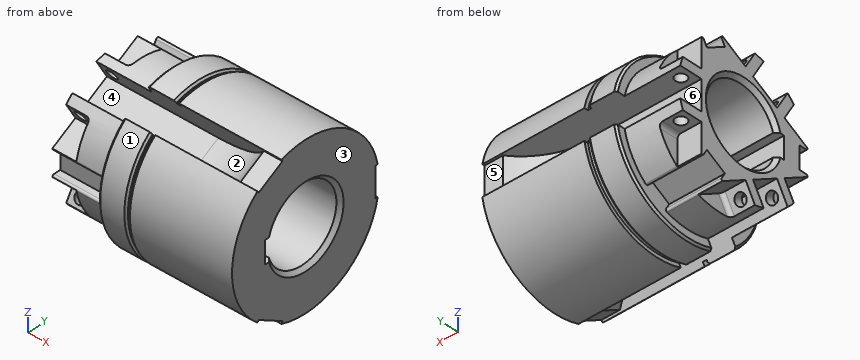
from build123d import *

# Parameters (mm, degrees)
CUT_EXTRUDE1_DEPTH       = 8
CIRPATTERN1_COUNT        = 3
CUT_EXTRUDE2_DEPTH       = 13
FILLET1_R                = 2
CUT_EXTRUDE3_REACH       = 125.655
SKETCH6_R                = 3
CIRPATTERN2_COUNT        = 3
FILLET1_OF_CIRPATTERN2_R = 2
CUT_EXTRUDE4_DEPTH       = 30
FILLET2_R                = 1
CIRPATTERN3_COUNT        = 3
FILLET2_OF_CIRPATTERN3_R = 1
CUT_EXTRUDE5_REACH       = 130.22
SKETCH9_W                = 102
SKETCH9_H                = 12
CHAMFER2_SIZE            = 2
CHAMFER3_SIZE            = 1


with BuildPart() as part:
    # Sketch1 → Revolve1 (revolve)
    with BuildSketch(Plane.XY, mode=Mode.PRIVATE) as revolve1_sk:
        Polygon((0, 20), (0, 42.5), (-55, 42.5), (-55, 40.5), (-57, 40.5), (-57, 42.5), (-72, 42.5), (-72, 37.6), (-102, 37.6), (-102, 20), align=None)
    revolve(revolve1_sk.sketch.rotate(Axis((-534.701035213, 0, 0), (1, 0, 0)), 90), axis=Axis((-534.701035213, 0, 0), (1, 0, 0)))

    # Sketch3 → Cut-Extrude1 (cut, symmetric)
    with BuildSketch(Plane.XY):
        with BuildLine():
            Line((-102, 24.5), (-42, 24.5))
            ThreePointArc((-42, 24.5), (-24.11145618, 28.72291236), (-10, 40.5))
            Line((-10, 40.5), (0, 40.5))
            Line((0, 40.5), (0, 42.5))
            Line((0, 42.5), (-55, 42.5))
            Line((-55, 42.5), (-55, 40.5))
            Line((-55, 40.5), (-57, 40.5))
            Line((-57, 40.5), (-57, 42.5))
            Line((-57, 42.5), (-72, 42.5))
            Line((-72, 42.5), (-72, 37.6))
            Line((-72, 37.6), (-102, 37.6))
            Line((-102, 37.6), (-102, 24.5))
        make_face()
    cut_extrude1 = extrude(amount=CUT_EXTRUDE1_DEPTH, both=True, mode=Mode.SUBTRACT)

    # CirPattern1: Cut-Extrude1 ×3 about axis
    cirpattern1_axis = Axis((0, 0, 0), (1, 0, 0))
    for i in range(1, CIRPATTERN1_COUNT):
        add(cut_extrude1.rotate(cirpattern1_axis, i * 360 / CIRPATTERN1_COUNT), mode=Mode.SUBTRACT)

    # Sketch4 → Cut-Extrude2 (cut)
    with BuildSketch(Plane.ZY.offset(102)):
        with BuildLine():
            Line((-13, 35.281156444), (-13, 24.5))
            Line((-13, 24.5), (-28.522096697, 24.5))
            ThreePointArc((-28.522096697, 24.5), (-21.449462979, 30.881718506), (-13, 35.281156444))
        make_face()
        with BuildLine():
            Line((13, 35.281156444), (13, 24.5))
            Line((13, 24.5), (28.522096697, 24.5))
            ThreePointArc((28.522096697, 24.5), (21.449462979, 30.881718506), (13, 35.281156444))
        make_face()
    cut_extrude2 = extrude(amount=-CUT_EXTRUDE2_DEPTH, mode=Mode.SUBTRACT)

    # Fillet1
    fillet1_edges = [part.edges().sort_by_distance(p)[0] for p in [
        (-89, 29.890578222, -13),
        (-89, 29.890578222, 13),
    ]]
    fillet(fillet1_edges, radius=FILLET1_R)

    # Cut-Extrude3: up to this face of the body (flat: up to its plane)
    cut_extrude3_end = Plane(part.part.faces().sort_by_distance((-96.5, 29.890578222, -13))[0])
    # Sketch6 → Cut-Extrude3 (cut, up to the picked face)
    with BuildSketch(Plane.XY.offset(13), mode=Mode.PRIVATE) as cut_extrude3_sk1:
        with Locations((-96.5, 30.5)):
            Circle(SKETCH6_R)
    cut_extrude3_tool1 = split(extrude(cut_extrude3_sk1.sketch, amount=-CUT_EXTRUDE3_REACH, mode=Mode.PRIVATE), bisect_by=cut_extrude3_end, keep=Keep.BOTH, mode=Mode.PRIVATE)
    cut_extrude3 = cut_extrude3_tool1.solids().sort_by(Axis((-96.5, 30.5, 13), (0, 0, -1)))[0]
    add(cut_extrude3, mode=Mode.SUBTRACT)

    # CirPattern2: Cut-Extrude2, Cut-Extrude3 ×3 about axis
    cirpattern2_axis = Axis((0, 0, 0), (1, 0, 0))
    add([cut_extrude2.rotate(cirpattern2_axis, i * 360 / CIRPATTERN2_COUNT) for i in range(1, CIRPATTERN2_COUNT)], mode=Mode.SUBTRACT)
    add([cut_extrude3.rotate(cirpattern2_axis, i * 360 / CIRPATTERN2_COUNT) for i in range(1, CIRPATTERN2_COUNT)], mode=Mode.SUBTRACT)

    # Fillet1 of CirPattern2
    fillet1_of_cirpattern2_edges = [part.edges().sort_by_distance(p)[0] for p in [
        (-89, -3.686958862, 32.386000074),
        (-89, -26.20361936, 19.386000074),
        (-89, -26.20361936, -19.386000074),
        (-89, -3.686958862, -32.386000074),
    ]]
    fillet(fillet1_of_cirpattern2_edges, radius=FILLET1_OF_CIRPATTERN2_R)

    # Sketch7 → Cut-Extrude4 (cut)
    with BuildSketch(Plane.ZY.offset(102)):
        with BuildLine():
            Line((-6, -37.118189611), (-6, -32.3))
            Line((-6, -32.3), (6, -32.3))
            Line((6, -32.3), (6, -37.118189611))
            ThreePointArc((6, -37.118189611), (0, -37.6), (-6, -37.118189611))
        make_face()
    cut_extrude4 = extrude(amount=-CUT_EXTRUDE4_DEPTH, mode=Mode.SUBTRACT)

    # Fillet2
    fillet2_edges = [part.edges().sort_by_distance(p)[0] for p in [
        (-87, -37.118189611, 6),
        (-87, -37.118189611, -6),
    ]]
    fillet(fillet2_edges, radius=FILLET2_R)

    # CirPattern3: Cut-Extrude4 ×3 about axis
    cirpattern3_axis = Axis((0, 0, 0), (1, 0, 0))
    for i in range(1, CIRPATTERN3_COUNT):
        add(cut_extrude4.rotate(cirpattern3_axis, i * 360 / CIRPATTERN3_COUNT), mode=Mode.SUBTRACT)

    # Fillet2 of CirPattern3
    fillet2_of_cirpattern3_edges = [part.edges().sort_by_distance(p)[0] for p in [
        (-87, 13.362942383, -35.145295146),
        (-87, 23.755247228, -29.145295146),
        (-87, 23.755247228, 29.145295146),
        (-87, 13.362942383, 35.145295146),
    ]]
    fillet(fillet2_of_cirpattern3_edges, radius=FILLET2_OF_CIRPATTERN3_R)

    # Sketch9 → Cut-Extrude5 (cut, up to next)
    with BuildSketch(Plane(origin=(0, -23.3, 0), x_dir=(1, 0, 0), z_dir=(0, 1, 0)), mode=Mode.PRIVATE) as cut_extrude5_sk1:
        with Locations((-51, 0)):
            Rectangle(SKETCH9_W, SKETCH9_H)
    cut_extrude5_tool1 = extrude(cut_extrude5_sk1.sketch, amount=CUT_EXTRUDE5_REACH, mode=Mode.PRIVATE) & part.part
    add(cut_extrude5_tool1.solids().sort_by_distance((-51, -23.3, 0))[0], mode=Mode.SUBTRACT)

    # Chamfer2
    chamfer2_edges = [part.edges().sort_by_distance(p)[0] for p in [
        (0, 20, 0),
        (-102, 20, 0),
    ]]
    chamfer(chamfer2_edges, length=CHAMFER2_SIZE)

    # Chamfer3
    chamfer3_edges = [part.edges().sort_by_distance(p)[0] for p in [
        (-72, -42.5, 0),
        (-72, 21.25, 36.806079661),
        (-57, -42.5, 0),
        (-57, 21.25, 36.806079661),
        (-72, 21.25, -36.806079661),
        (-57, 21.25, -36.806079661),
    ]]
    chamfer(chamfer3_edges, length=CHAMFER3_SIZE)


solid = part.part
The model under review builds one solid part; all positions refer to its coordinate system, in mm. Face numbers are marked on the shaded views. A direction names the side the tool comes from. Give positions to 0.01 mm unless a question says otherwise; leave off trailing zeros. Write each loop counter-clockwise with the first axis right and the second up, starting at its lowest first coordinate (ties: lowest second). Pieces come first, ordered by that corner, then holes. Notation, with made-up numbers: M -9.75,-2.75 L 24.25,-2.75 A31 cw 24.25,26.25 Z; hole C 86,25 d8. An arc over 180 degrees is marked long. One line per question, with ' | ' between items. Start each with the question number.
Item 1: Wall thickness on line 1 (Z direction, x = -60, y = 0); line 2 (Y direction, x = -96.5, z = -11.8); line 3 (Z direction, x = -24.5, y = -9): over which ranges is each line inside the solid? List them lowest first. Write a range as from..to.
Item 2: We need section A-A on z = 0. Write out the cut boundary in (x, y), plus the area to 3 significant figures.
Item 3: For the marked faces 4, 5 and 6, list the 3-axis set-ups (+Z, -Z, +X, -X, +Y, -Y) from which the entire face can be reached by the end or side of a thin tool; tool diameter is ignored.
Item 4: We need section B-B on x = -50.5. Write out the cut boundary in (y, z).
Item 5: We need section C-C on x = -96.5. Give the number of separate pieces and of enclosed holes in the cut face, plus the area to 3 significant figures.
Item 6: Draft analysis for pull direction X (two halves, no side actions). For the marked faces 1, 2 and 3, state which applies: released by +X, released by -X, zero draft, split by the parting line, or undercut.
Item 7: For pin 1 (8.5 mm diameter, centred on x = -96, y = 30.5, fed in from -Z); pin 2 (4.5 mm diameter, centred on y = 1, z = 34, fed in from -X); pin 3 (1.5 mm diameter, centred on x = -48, y = -13, fed in from -Z); pin 4 (1.5 mm diameter, centred on y = -12.5, z = -12, fed in from -X), all flat-tipped, find the tip position at first contact; note any pin that passes through.
Results found:
1) line 1: z = -42.5..-20, 20..42.5 | line 2: y = -28.56..-16.15, 16.15..27.5, 33.5..35.7 | line 3: z = -41.54..-31.59, -27.75..-17.86, 17.86..27.75, 31.59..41.54
2) outline: M -102,-32.3 L -72,-32.3 L -72,-41.5 L -71,-42.5 L -58,-42.5 L -57,-41.5 L -57,-40.5 L -55,-40.5 L -55,-42.5 L 0,-42.5 L 0,-23.3 L -102,-23.3 Z; M -102,22 L -100,20 L -2,20 L 0,22 L 0,40.5 L -10,40.5 A40 cw -42,24.5 L -102,24.5 Z | area: 2,420 mm2
3) face 4: -X | face 5: +X, -X, +Y | face 6: -X, +Y
4) outline: M -27.8,-32.15 L -19.18,-17.22 L -5.32,-25.22 L -13.94,-40.15 A42.5 ccw 41.74,-8 L 24.5,-8 L 24.5,8 L 41.74,8 A42.5 ccw -13.94,40.15 L -5.32,25.22 L -19.18,17.22 L -27.8,32.15 A42.5 ccw Z; hole M -23.3,-6 L -19.08,-6 A20 ccw long -19.08,6 L -23.3,6 Z
5) separate pieces: 7 | enclosed holes: 1 | area: 1,570 mm2
6) face 1: zero draft | face 2: released by -X | face 3: released by +X
7) pin 1: stops at z = -13 | pin 2: stops at x = -89 | pin 3: stops at z = -40.7 | pin 4: passes through
